Autodesk Inventor part; units mm, degrees
ref_plane "YZ Plane" through (0, 0, 0) normal (1, 0, 0) x (0, 1, 0)
ref_plane "XZ Plane" through (0, 0, 0) normal (0, 1, 0) x (-1, 0, 0)
ref_plane "XY Plane" through (0, 0, 0) normal (0, 0, 1) x (1, 0, 0)
sketch "スケッチ1" plane through (0, 0, 0) normal (0, 0, 1) x (1, 0, 0)
  circle A0 centre (0, 0) radius 27.25
  line L0 (17.5, 17.5) -> (-17.5, 17.5)
  line L1 (-17.5, 17.5) -> (-17.5, -17.5)
  line L2 (-17.5, -17.5) -> (17.5, -17.5)
  line L3 (17.5, -17.5) -> (17.5, 17.5)
  line L4 (17.5, 17.5) -> (-17.5, -17.5) construction
  line L5 (-17.5, 17.5) -> (17.5, -17.5) construction
  line L6 (1, 17.5) -> (-1, 17.5)
  line L7 (-1, 17.5) -> (-1, -17.5)
  line L8 (-1, -17.5) -> (1, -17.5)
  line L9 (1, -17.5) -> (1, 17.5)
  line L10 (1, 17.5) -> (-1, -17.5) construction
  line L11 (-1, 17.5) -> (1, -17.5) construction
  point P0 (1, -17.5)
  point P1 (1, 17.5)
  point P2 (-1, 17.5)
  point P3 (-1, -17.5)
  dimension "d0" = 54.5
  dimension "d6" = 35
  dimension "d107" = 2
  dimension "d108" = 35
extrude "押し出し1" add sketch "スケッチ1" against normal blind 1 contours A0 | L9 L2 L7 L0
sketch "スケッチ2" plane through (0, 0, 0) normal (0, 0, 1) x (1, 0, 0)
  line L0 (0, 42.4511) -> (0, -37.5489)
  line L1 (38.0038, 0) -> (-41.9962, 0)
  line L2 (27.25, 42.0143) -> (27.25, -37.9857)
  circle A0 centre (0, 0) radius 27.25
  line L3 (17.5, 17.5) -> (17.5, -17.5)
  line L4 (19.25, 25) -> (27.25, 25)
  line L5 (27.25, 25) -> (27.25, -25)
  line L6 (27.25, -25) -> (19.25, -25)
  line L7 (19.25, -25) -> (19.25, 25)
  line L8 (19.25, 25) -> (27.25, -25) construction
  line L9 (27.25, 25) -> (19.25, -25) construction
  point P0 (17.5, 0)
  point P1 (23.25, 0)
  point P2 (19.25, 0)
  point P3 (27.25, 0)
  dimension "d13" = 9.75
  dimension "d14" = 8
  dimension "d15" = 50
  dimension "d19" = 54.5
  dimension "d110" = 1.75
extrude "押し出し2" cut sketch "スケッチ2" against normal blind 10 contours L7 L4 L2 A0 | A0 L1 L7 picked at (20.3822, 11.481)
mirror "ミラー1" about plane through (0, 0, 0) normal (1, 0, 0) of "押し出し2"
sketch "スケッチ8" plane through (0, 0, 0) normal (0, 0, 1) x (1, 0, 0)
  circle A0 centre (0, 0) radius 22.375
  circle A1 centre (0, 0) radius 27.25
  line L0 (0, 31.1603) -> (0, -30.8706)
  point P0 (0, 0)
  point P1 (0, 22.375)
  point P2 (0, -22.375)
  dimension "d112" = 44.75
  dimension "d113" = 54.5
hole "穴5" at (0, 22.375, 0) at (0, -22.375, 0) direction (0, 0, -1) diameter 6.6 end through all
properties part number "Part3_A_Y" material "鋼、軟鋼"
For this review, take the finished solid that the model builds, in its own axes (mm). Coordinates: 2 decimals unless noted, no trailing zeros. Loops run counter-clockwise (first coordinate to the right, second up) from the corner with the lowest first, then second, coordinate; pieces in that order, holes last. Notation, with made-up numbers: (-36, -35) - (-26, -35) arc R16 cw to (-26, -20) - close; hole circle Ø2 at (-34.75, 2.5). An arc over 180 degrees is marked (long way). Return JSON: item names as keys, results as strings.
Item 1: Take a section at B-B (x = 0). Give the boundary of the cut face in (y, z) (3 decimals), then the cut area to 3 significant figures.
Determined:
{"outline": "(-27.25, -1) - (-25.675, -1) - (-25.675, 0) - (-27.25, 0) - close; (-19.075, -1) - (19.075, -1) - (19.075, 0) - (-19.075, 0) - close; (25.675, -1) - (27.25, -1) - (27.25, 0) - (25.675, 0) - close", "area": "41.3 mm2"}
Item 2: Take a section at A-A (y = 13). Give the boundary of the cut face in (x, z), then the cut area to 3 significant figures.
Determined:
{"outline": "(-19.25, -1) - (-17.5, -1) - (-17.5, 0) - (-19.25, 0) - close; (-1, -1) - (1, -1) - (1, 0) - (-1, 0) - close; (17.5, -1) - (19.25, -1) - (19.25, 0) - (17.5, 0) - close", "area": "5.50 mm2"}
Item 3: For line 1 (X direction, y = 6, z = -0.8); line 2 (Y direction, x = 0, z = -0.75) (3 decimals); line 3 (X direction, y = -4, z = -0.65), list the stretches that pass through material, from the lowest coordinate up.
Determined:
{"line 1": "x = -19.25 to -17.5, -1 to 1, 17.5 to 19.25", "line 2": "y = -27.25 to -25.675, -19.075 to 19.075, 25.675 to 27.25", "line 3": "x = -26.95 to -17.5, -1 to 1, 17.5 to 26.95"}
Item 4: Take a section at D-D (y = -22). Give the boundary of the cut face in (x, z), then the cut area to 3 significant figures.
Determined:
{"outline": "(-16.08, -1) - (-3.28, -1) - (-3.28, 0) - (-16.08, 0) - close; (3.28, -1) - (16.08, -1) - (16.08, 0) - (3.28, 0) - close", "area": "25.6 mm2"}
Item 5: Mouldability with a two-part tool opening along Y and no side actions: class faces 1 (the cylindrical face through (1.264, -25.423, -0.507)), 2 (the cylindrical face through (-0.599, -27.243, -0.493)), 3 (the flat face through (0, 0, -1)), 4 (the cylindrical face through (1.264, 19.327, -0.507)) as pulls with the +Y half, pulls with the -Y half, needs draft (parallel to the pull), parting line crosses it, or undercut.
Determined:
{"face 1": "undercut", "face 2": "pulls with the -Y half", "face 3": "needs draft", "face 4": "undercut"}
Item 6: Take a section at C-C (z = -0.45). Give the boundary of the cut face in (x, y) (3 decimals).
Determined:
{"outline": "(-27.25, 0) arc R27.25 ccw to (27.25, 0) - (19.25, 0) - (19.25, 19.287) arc R27.25 ccw to (-19.25, 19.287) - (-19.25, 0) - close; hole (-17.5, -17.5) - (-1, -17.5) - (-1, 17.5) - (-17.5, 17.5) - close; hole circle Ø6.6 at (0, -22.375); hole circle Ø6.6 at (0, 22.375); hole (1, -17.5) - (17.5, -17.5) - (17.5, 17.5) - (1, 17.5) - close"}
Item 7: Insertion check: pin 1 (0.5 mm diameter, centred on y = -1.5, z = -0.5, fed in from +X); pin 2 (0.5 mm diameter, centred on y = -8, z = -0.5, fed in from -X); pin 3 (0.5 mm diameter, centred on y = -8.5, z = -0.5, fed in from -X); pin 4 (8.5 mm diameter, centred on x = 0, y = -22.375, fed in from +Z). Each pin has a flat end and moves straight along its axis. Give the tip position at first contact, or say it passes through.
Determined:
{"pin 1": "stops at x = 27.22", "pin 2": "stops at x = -26.12", "pin 3": "stops at x = -25.97", "pin 4": "stops at z = 0"}
